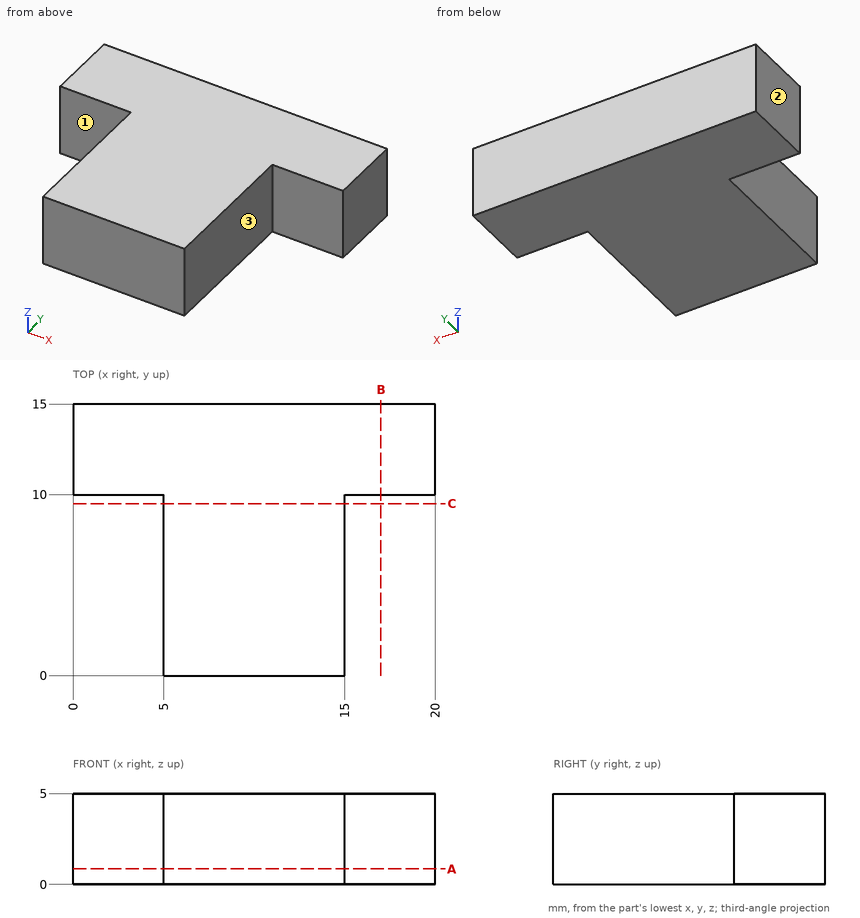
Here's the drawing with two shaded views (mm, measured from the low corner). I have some questions. A direction names the side the tool comes from. Round coordinates to 2 decimals unless told otherwise and drop trailing zeros. Write each loop counter-clockwise with the first axis right and the second up, starting at its lowest first coordinate (ties: lowest second). Pieces come first, ordered by that corner, then holes.
(1) Suppose I cut it at A-A on z = 0.85. Write out the boundary of the cut face in (x, y), and give its area (3 significant figures).
Findings below:
outline: (0, 10) - (5, 10) - (5, 0) - (15, 0) - (15, 10) - (20, 10) - (20, 15) - (0, 15) - close
area: 200 mm2
(2) Which directions (+Z, -Z, +X, -X, +Y, -Y) give clear straight access to the entire face, cutting with the end or side of a thin tool? Please do the marked faces 1, 2 and 3.
Findings below:
face 1: +Z, -Z, -X, -Y
face 2: +Z, -Z, -X, +Y, -Y
face 3: +Z, -Z, +X, -Y
(3) Suppose I cut it at C-C on y = 9.5. Write out the boundary of the cut face in (x, z).
Findings below:
outline: (5, 0) - (15, 0) - (15, 5) - (5, 5) - close
(4) Suppose I cut it at B-B on x = 17. Write out the boundary of the cut face in (y, z).
Findings below:
outline: (10, 0) - (15, 0) - (15, 5) - (10, 5) - close
(5) For pin 1 (1.5 mm diameter, centred on x = 1.5, z = 3, fed in from -Y); pin 2 (1 mm diameter, centred on y = 1.5, z = 0.5, fed in from -X), each with a flat end and sliding along its axis, tell me the tip position at first contact or that it passes through.
Findings below:
pin 1: stops at y = 10
pin 2: stops at x = 5
(6) If I drill on probe 1 along X at (y, z) = (6.5, 4.35); probe 2 along Y at (x, z) = (1.75, 3.1), over which ranges is the centre line in solid material (lowest first)?
Findings below:
probe 1: x = 5 to 15
probe 2: y = 10 to 15
